Part model, mm, in its own coordinate system. Give positions to 0.01 mm unless a question says otherwise; leave off trailing zeros. Order: outer loops, then holes, each group sorted by start corner. A loop starts at its lowest first (then second) coordinate and runs counter-clockwise, first axis right, second up. Notation, with made-up numbers: (-12.75, 57.5) -> (7.25, 57.5) arc R16 cw to (7.25, 61.5) -> close; hole circle Ø3 at (-23.5, 32). An arc over 180 degrees is marked (long way). Write item = value, one per line. Start each with the question number.
Item 1: Band-saw the part on C-C on y = 134. Write the cut outline in (x, z).
Item 2: Band-saw the part on B-B on x = 202. Write the cut outline in (y, z), plus the area to 3 significant figures.
Item 3: Band-saw the part on A-A on z = -3.5. Write the cut outline in (x, y).
Item 4: Drill centre lines: line 1 along Y through (x, z) = (199, -2.5); line 2 along Y through (x, z) = (-117, 3); line 3 along X through (y, z) = (137.5, -3). Where is each one in solid material? Low to high.
```python
from build123d import *

# Parameters (mm, degrees)
BOSS_EXTRUDE1_DEPTH = 5


with BuildPart() as part:
    # Sketch1 → Boss-Extrude1 (new body, symmetric)
    with BuildSketch(Plane.XY):
        with BuildLine():
            Line((-190, 153.262074111), (290, 153.262074111))
            ThreePointArc((290, 153.262074111), (297.071067812, 150.333141922), (300, 143.262074111))
            Line((300, 143.262074111), (300, 123.262074111))
            ThreePointArc((300, 123.262074111), (297.071067812, 116.191006299), (290, 113.262074111))
            Line((290, 113.262074111), (-190, 113.262074111))
            ThreePointArc((-190, 113.262074111), (-197.071067812, 116.191006299), (-200, 123.262074111))
            Line((-200, 123.262074111), (-200, 143.262074111))
            ThreePointArc((-200, 143.262074111), (-197.071067812, 150.333141922), (-190, 153.262074111))
        make_face()
        with BuildLine():
            Line((-169.867316387, 142.322613738), (270.03251135, 141.702162641))
            ThreePointArc((270.03251135, 141.702162641), (280.018397045, 131.68806823), (270.004302633, 121.702182535))
            Line((270.004302633, 121.702182535), (-169.895525104, 122.322633632))
            ThreePointArc((-169.895525104, 122.322633632), (-179.881410799, 132.336728043), (-169.867316387, 142.322613738))
        make_face(mode=Mode.SUBTRACT)
    extrude(amount=BOSS_EXTRUDE1_DEPTH, both=True)


solid = part.part
```
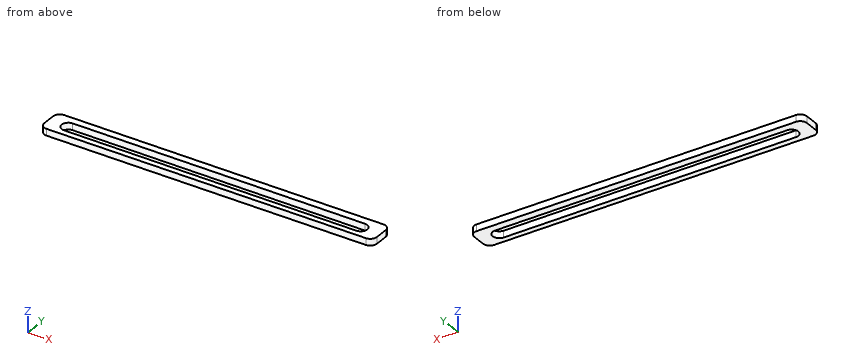
Values found:
q1.outline = (-200, -5) -> (-179.74, -5) -> (-179.74, 5) -> (-200, 5) -> close; (279.75, -5) -> (300, -5) -> (300, 5) -> (279.75, 5) -> close
q2.outline = (113.26, -5) -> (121.8, -5) -> (121.8, 5) -> (113.26, 5) -> close; (141.8, -5) -> (153.26, -5) -> (153.26, 5) -> (141.8, 5) -> close
q2.area = 200 mm^2
q3.outline = (-200, 123.26) arc R10 ccw to (-190, 113.26) -> (290, 113.26) arc R10 ccw to (300, 123.26) -> (300, 143.26) arc R10 ccw to (290, 153.26) -> (-190, 153.26) arc R10 ccw to (-200, 143.26) -> close; hole (-169.9, 122.32) -> (270, 121.7) arc R10 ccw to (270.03, 141.7) -> (-169.87, 142.32) arc R10 ccw to start
q4.line_1 = 113.26 to 121.8, 141.8 to 153.26
q4.line_2 = 113.26 to 122.25, 142.25 to 153.26
q4.line_3 = -200 to -178.44, 278.17 to 300
